from build123d import *

# Parameters (mm, degrees)
F0_R     = 48.2949752594
F1_DEPTH = 104.394
F2_R     = 14.4852813742
F3_T     = -4
F6_DEPTH = 8.1


# Not quite as in the source:
# - a feature of the source that left no trace in its solid (it failed there, or was rolled back) is left out


with BuildPart() as f1:
    # F0 (on Top) → F1 (new body)
    with BuildSketch(Plane.XY):
        with Locations((6.398510754, 6.8632753311)):
            Circle(F0_R)
    extrude(amount=F1_DEPTH)

    # F2
    f2_edges = [f1.edges().sort_by_distance(p)[0] for p in [
        (-41.896465, 6.863275, 0),
    ]]
    fillet(f2_edges, radius=F2_R)

    # F3
    f3_openings = [f1.faces().sort_by_distance(p)[0] for p in [
        (6.398511, 6.863275, 104.394),
    ]]
    offset(amount=F3_T, openings=f3_openings)

    # F5 (on Right) → F6 (join, symmetric)
    with BuildSketch(Plane.YZ):
        with BuildLine():
            Line((-38.8429239392, 77.0174632754), (-38.8429239392, 81.8370801914))
            ThreePointArc((-38.8429239392, 81.8370801914), (-88.478602233, 55.4130888204), (-41.5783710778, 24.392189458))
            Line((-41.5783710778, 24.392189458), (-41.5783710778, 30.7706389778))
            Line((-41.5783710778, 30.7706389778), (-44.6209337434, 30.6963794891))
            ThreePointArc((-44.6209337434, 30.6963794891), (-81.5156325698, 53.8569213822), (-44.6209337434, 77.0174632754))
            Line((-44.6209337434, 77.0174632754), (-38.8429239392, 77.0174632754))
        make_face()
    extrude(amount=F6_DEPTH, both=True)


solid = f1.part
The listing builds one solid part. Answer for the finished solid, in the listing's coordinates (mm). A direction names the side the tool comes from. Give positions to 0.01 mm unless a question says otherwise; leave off trailing zeros. Loops run counter-clockwise (first coordinate to the right, second up) from the corner with the lowest first, then second, coordinate; pieces in that order, holes last.
Item 1: Each of these flat-tipped pins is pushed along its axis until it touches: pin 1 Ø6 at (y, z) = (35.5, 88) entering from -X; pin 2 Ø3 at (x, y) = (28.5, -9) entering from -Z; pin 3 Ø8 at (y, z) = (-59, 23.5) entering from -X; pin 4 Ø2 at (x, y) = (40.5, 26) entering from -Z. Where does it stop, or does it pass through?
Derived:
pin 1: stops at x = -34.53
pin 2: stops at z = 0
pin 3: stops at x = -8.1
pin 4: stops at z = 0.65
Item 2: Determine the mould class of faces 1 (the cylindrical face through (0.111, 54.747, 58.81)), 2 (the cylindrical face through (-3.2, -36.38, 58.81)), 3 (the cylindrical face through (0.113, -81.505, 53.13)) for opening direction X: +X half, -X half, draft (parallel to the pull), parting line (faces both ways), or undercut.
Derived:
face 1: parting line
face 2: undercut
face 3: draft
Item 3: A cutting plane is placed at A-A (z = 66). Give the vertices of the cut face in (x, y), then the cut area to 3 significant figures.
Derived:
outline: circle Ø96.59 at (6.4, 6.86); (-8.1, -86.18) - (8.1, -86.18) - (8.1, -78.47) - (-8.1, -78.47) - close; hole circle Ø88.59 at (6.4, 6.86)
area: 1,290 mm2
Item 4: A cutting plane is placed at B-B (y = -74). Give the vertices of the cut face in (x, z), then the cut area to 3 significant figures.
Derived:
outline: (-8.1, 26.67) - (8.1, 26.67) - (8.1, 35.69) - (-8.1, 35.69) - close; (-8.1, 72.02) - (8.1, 72.02) - (8.1, 81.04) - (-8.1, 81.04) - close
area: 292 mm2
Item 5: A tool of negligible diameter and unlimited length cuts with its end or side. For faces 4 (the flat face through (0, -41.578, 28)), 5 (the flat face through (-8.1, -82, 56)), 6 (the flat face through (6, 7, 4)), 7 (the flat face through (8.1, -83, 54)), from which of +Z, -Z, +X, -X, +Y, -Y can it reach the whole face along a straight path? Write none if from no direction.
Derived:
face 4: -Z, +X, -X
face 5: +Z, -Z, -X, -Y
face 6: +Z
face 7: +Z, -Z, +X, -Y
Item 6: A cutting plane is placed at C-C (z = 53). Give the vertices of the cut face in (x, y).
Derived:
outline: circle Ø96.59 at (6.4, 6.86); (-8.1, -88.5) - (8.1, -88.5) - (8.1, -81.5) - (-8.1, -81.5) - close; hole circle Ø88.59 at (6.4, 6.86)
Item 7: Find the intervals of material crossed by line 1 along X through (y, z) = (8, 48.5); line 2 along Y through (x, z) = (-3.5, 13); line 3 along Y through (x, z) = (-14.5, 64), in increasing order.
Derived:
line 1: x = -41.88 to -37.88, 50.68 to 54.68
line 2: y = -40.33 to -36.2, 49.93 to 54.05
line 3: y = -36.68 to -32.19, 45.92 to 50.4
Item 8: A cutting plane is placed at D-D (y = -56.5). Give the vertices of the cut face in (x, z).
Derived:
outline: (-8.1, 21.15) - (8.1, 21.15) - (8.1, 28.15) - (-8.1, 28.15) - close; (-8.1, 79.56) - (8.1, 79.56) - (8.1, 86.57) - (-8.1, 86.57) - close
